Read the model definition and answer for the solid it produces. Units are mm, in the model's axes. A direction names the side the tool comes from. Coordinates: 2 decimals unless noted, no trailing zeros. Order: outer loops, then holes, each group sorted by start corner. A loop starts at its lowest first (then second) coordinate and runs counter-clockwise, first axis right, second up. Notation, with made-up numbers: M -8,54.25 L 5,54.25 A38 cw 5,92.25 Z; hole C -26,0 d10. An arc over 180 degrees is marked long. Write each question's results on one line, items separated by ' | '.
```python
from build123d import *

# Parameters (mm, degrees)
SKETCH2_R           = 3.55
BOSS_EXTRUDE1_DEPTH = 3.8
BOSS_EXTRUDE2_DEPTH = 1.4
SKETCH5_R           = 2.549999919
CUT_EXTRUDE1_DEPTH  = 2.5
BOSS_EXTRUDE3_DEPTH = 2.5
SKETCH6_R           = 1.4
CUT_EXTRUDE2_DEPTH  = 12.745554295
SKETCH7_R           = 0.6
CUT_EXTRUDE3_DEPTH  = 12.724676785


with BuildPart() as part:
    # Sketch2 → Boss-Extrude1 (new body)
    with BuildSketch(Plane.XY):
        Circle(SKETCH2_R)
    extrude(amount=-BOSS_EXTRUDE1_DEPTH)

    # Sketch4 → Boss-Extrude2 (add)
    with BuildSketch(Plane.XY.offset(-2.4)):
        with BuildLine():
            Line((2.776387215, 2.212277889), (10.622617722, 1.649999976))
            ThreePointArc((10.622617722, 1.649999976), (10.913548722, 0), (10.622617722, -1.649999976))
            Line((10.622617722, -1.649999976), (2.776387215, -2.212277889))
            ThreePointArc((2.776387215, -2.212277889), (3.549999952, 0), (2.776387215, 2.212277889))
        make_face()
    extrude(amount=-BOSS_EXTRUDE2_DEPTH)

    # Sketch5 → Cut-Extrude1 (cut)
    with BuildSketch(Plane.XY):
        Circle(SKETCH5_R)
    extrude(amount=-CUT_EXTRUDE1_DEPTH, mode=Mode.SUBTRACT)

    # Sketch3 → Boss-Extrude3 (add)
    with BuildSketch(Plane.XY):
        with BuildLine():
            Line((-0.244697916, 2.538232164), (0, 2.049999952))
            Line((0, 2.049999952), (0.244697916, 2.538232164))
            ThreePointArc((0.244697916, 2.538232164), (0, 2.549999919), (-0.244697916, 2.538232164))
        make_face()
        with BuildLine():
            Line((0.551635326, 2.489618054), (0.633484824, 1.949665813))
            Line((0.633484824, 1.949665813), (1.017078422, 2.338386424))
            ThreePointArc((1.017078422, 2.338386424), (0.787993311, 2.42519404), (0.551635326, 2.489618054))
        make_face()
        with BuildLine():
            Line((1.29397066, 2.197302783), (1.204959739, 1.6584848))
            Line((1.204959739, 1.6584848), (1.689900206, 1.90964313))
            ThreePointArc((1.689900206, 1.90964313), (1.498852346, 2.06299327), (1.29397066, 2.197302783))
        make_face()
        with BuildLine():
            Line((1.90964313, 1.689900206), (1.6584848, 1.204959739))
            Line((1.6584848, 1.204959739), (2.197302783, 1.29397066))
            ThreePointArc((2.197302783, 1.29397066), (2.06299327, 1.498852346), (1.90964313, 1.689900206))
        make_face()
        with BuildLine():
            Line((2.338386424, 1.017078422), (1.949665813, 0.633484824))
            Line((1.949665813, 0.633484824), (2.489618054, 0.551635326))
            ThreePointArc((2.489618054, 0.551635326), (2.42519404, 0.787993311), (2.338386424, 1.017078422))
        make_face()
        with BuildLine():
            Line((2.538232164, 0.244697916), (2.049999952, 0))
            Line((2.049999952, 0), (2.538232164, -0.244697916))
            ThreePointArc((2.538232164, -0.244697916), (2.549999919, 0), (2.538232164, 0.244697916))
        make_face()
        with BuildLine():
            Line((2.489618054, -0.551635326), (1.949665813, -0.633484824))
            Line((1.949665813, -0.633484824), (2.338386424, -1.017078422))
            ThreePointArc((2.338386424, -1.017078422), (2.42519404, -0.787993311), (2.489618054, -0.551635326))
        make_face()
        with BuildLine():
            Line((2.197302783, -1.29397066), (1.6584848, -1.204959739))
            Line((1.6584848, -1.204959739), (1.90964313, -1.689900206))
            ThreePointArc((1.90964313, -1.689900206), (2.06299327, -1.498852346), (2.197302783, -1.29397066))
        make_face()
        with BuildLine():
            Line((1.689900206, -1.90964313), (1.204959739, -1.6584848))
            Line((1.204959739, -1.6584848), (1.29397066, -2.197302783))
            ThreePointArc((1.29397066, -2.197302783), (1.498852346, -2.06299327), (1.689900206, -1.90964313))
        make_face()
        with BuildLine():
            Line((1.017078422, -2.338386424), (0.633484824, -1.949665813))
            Line((0.633484824, -1.949665813), (0.551635326, -2.489618054))
            ThreePointArc((0.551635326, -2.489618054), (0.787993311, -2.42519404), (1.017078422, -2.338386424))
        make_face()
        with BuildLine():
            Line((0.244697916, -2.538232164), (0, -2.049999952))
            Line((0, -2.049999952), (-0.244697916, -2.538232164))
            ThreePointArc((-0.244697916, -2.538232164), (0, -2.549999919), (0.244697916, -2.538232164))
        make_face()
        with BuildLine():
            Line((-0.551635326, -2.489618054), (-0.633484824, -1.949665813))
            Line((-0.633484824, -1.949665813), (-1.017078422, -2.338386424))
            ThreePointArc((-1.017078422, -2.338386424), (-0.787993311, -2.42519404), (-0.551635326, -2.489618054))
        make_face()
        with BuildLine():
            Line((-1.29397066, -2.197302783), (-1.204959739, -1.6584848))
            Line((-1.204959739, -1.6584848), (-1.689900206, -1.90964313))
            ThreePointArc((-1.689900206, -1.90964313), (-1.498852346, -2.06299327), (-1.29397066, -2.197302783))
        make_face()
        with BuildLine():
            Line((-1.90964313, -1.689900206), (-1.6584848, -1.204959739))
            Line((-1.6584848, -1.204959739), (-2.197302783, -1.29397066))
            ThreePointArc((-2.197302783, -1.29397066), (-2.06299327, -1.498852346), (-1.90964313, -1.689900206))
        make_face()
        with BuildLine():
            Line((-2.338386424, -1.017078422), (-1.949665813, -0.633484824))
            Line((-1.949665813, -0.633484824), (-2.489618054, -0.551635326))
            ThreePointArc((-2.489618054, -0.551635326), (-2.42519404, -0.787993311), (-2.338386424, -1.017078422))
        make_face()
        with BuildLine():
            Line((-2.538232164, -0.244697916), (-2.049999952, 0))
            Line((-2.049999952, 0), (-2.538232164, 0.244697916))
            ThreePointArc((-2.538232164, 0.244697916), (-2.549999919, 0), (-2.538232164, -0.244697916))
        make_face()
        with BuildLine():
            Line((-2.489618054, 0.551635326), (-1.949665813, 0.633484824))
            Line((-1.949665813, 0.633484824), (-2.338386424, 1.017078422))
            ThreePointArc((-2.338386424, 1.017078422), (-2.42519404, 0.787993311), (-2.489618054, 0.551635326))
        make_face()
        with BuildLine():
            Line((-2.197302783, 1.29397066), (-1.6584848, 1.204959739))
            Line((-1.6584848, 1.204959739), (-1.90964313, 1.689900206))
            ThreePointArc((-1.90964313, 1.689900206), (-2.06299327, 1.498852346), (-2.197302783, 1.29397066))
        make_face()
        with BuildLine():
            Line((-1.689900206, 1.90964313), (-1.204959739, 1.6584848))
            Line((-1.204959739, 1.6584848), (-1.29397066, 2.197302783))
            ThreePointArc((-1.29397066, 2.197302783), (-1.498852346, 2.06299327), (-1.689900206, 1.90964313))
        make_face()
        with BuildLine():
            Line((-1.017078422, 2.338386424), (-0.633484824, 1.949665813))
            Line((-0.633484824, 1.949665813), (-0.551635326, 2.489618054))
            ThreePointArc((-0.551635326, 2.489618054), (-0.787993311, 2.42519404), (-1.017078422, 2.338386424))
        make_face()
    extrude(amount=-BOSS_EXTRUDE3_DEPTH)

    # Sketch6 → Cut-Extrude2 (cut, through all)
    with BuildSketch(Plane.XY.offset(-2.5)):
        Circle(SKETCH6_R)
    extrude(amount=-CUT_EXTRUDE2_DEPTH, mode=Mode.SUBTRACT)

    # Sketch7 → Cut-Extrude3 (cut, through all)
    with BuildSketch(Plane.XY.offset(-2.4)):
        with Locations((8.5405208, 0)):
            Circle(SKETCH7_R)
    extrude(amount=-CUT_EXTRUDE3_DEPTH, mode=Mode.SUBTRACT)


solid = part.part
```
(1) The mould has two halves that part along X. Classify faces 3 (the cylindrical face through (-1.4, 0.06, -3.14)), 4 (the flat face through (0.74, -2.32, 0)), 5 (the cylindrical face through (10.913, 0.024, -3.09)): pulls with the +X half, pulls with the -X half, needs draft (parallel to the pull), parting line crosses it, or undercut.
Conclusion:
face 3: undercut | face 4: needs draft | face 5: pulls with the +X half
(2) The part is cut by section B-B, the plane y = 3. Write down the section's boundary in (x, z).
Conclusion:
outline: M -1.9,-3.8 L 1.9,-3.8 L 1.9,0 L -1.9,0 Z
(3) Straight lines are drawn through the part: line 1 (Y direction, x = 0, z = -2.95); line 2 (X direction, y = -2.25, z = -0.2); line 3 (Y direction, x = 0.5, z = -1). For each, find the intervals that lie inside material, in ascending order.
Conclusion:
line 1: -3.55 to -1.4, 1.4 to 3.55 | line 2: -2.75 to -1.2, -0.93 to -0.59, -0.1 to 0.1, 0.59 to 0.93, 1.2 to 2.75 | line 3: -3.51 to -2.5, 2.5 to 3.51
(4) The part is cut by section A-A, the plane x = 7.5. Write down the section's boundary in (y, z), then the cut area to 3 significant figures.
Conclusion:
outline: M -1.87,-3.8 L 1.87,-3.8 L 1.87,-2.4 L -1.87,-2.4 Z | area: 5.25 mm²
(5) For faces 1 (the flat face through (4, 0, -3.8)), 2 (the cylindrical face through (-3.547, 0.156, -1.873)), determine the directions among +Z, -Z, +X, -X, +Y, -Y from which every point of the face is accessible in a straight line to the end or side of a thin tool.
Conclusion:
face 1: -Z, +X, -X, +Y, -Y | face 2: +Z
(6) Given pin 1 (1.1 mm diameter, centred on x = 8.54, y = 0, fed in from +Z), flat-ended and moving along its own axis, determine where the tip first touches the part or whether it passes through.
Conclusion:
pin 1: through
